```python
from build123d import *

# Parameters (mm, degrees)
SKETCH_1_W      = 1620
SKETCH_1_H      = 1620
SKETCH_1_W_2    = 500
SKETCH_1_H_2    = 500
EXTRUDE_1_DEPTH = 0.1


with BuildPart() as part:
    # 草图1 → 凸台-拉伸1 (new body)
    with BuildSketch(Plane(origin=(0, 0, 0), x_dir=(0, 0, -1), z_dir=(1, 0, 0))):
        Rectangle(SKETCH_1_W, SKETCH_1_H)
        with Locations((-540, 540)):
            Rectangle(SKETCH_1_W_2, SKETCH_1_H_2, mode=Mode.SUBTRACT)
        with Locations((0, 540)):
            Rectangle(SKETCH_1_W_2, SKETCH_1_H_2, mode=Mode.SUBTRACT)
        with Locations((540, 540)):
            Rectangle(SKETCH_1_W_2, SKETCH_1_H_2, mode=Mode.SUBTRACT)
        with Locations((540, 0)):
            Rectangle(SKETCH_1_W_2, SKETCH_1_H_2, mode=Mode.SUBTRACT)
        Rectangle(SKETCH_1_W_2, SKETCH_1_H_2, mode=Mode.SUBTRACT)
        with Locations((-540, 0)):
            Rectangle(SKETCH_1_W_2, SKETCH_1_H_2, mode=Mode.SUBTRACT)
        with Locations((-540, -540)):
            Rectangle(SKETCH_1_W_2, SKETCH_1_H_2, mode=Mode.SUBTRACT)
        with Locations((0, -540)):
            Rectangle(SKETCH_1_W_2, SKETCH_1_H_2, mode=Mode.SUBTRACT)
        with Locations((540, -540)):
            Rectangle(SKETCH_1_W_2, SKETCH_1_H_2, mode=Mode.SUBTRACT)
    extrude(amount=EXTRUDE_1_DEPTH)


solid = part.part
```
Source: CAD feature listing. Evaluate the final solid. Frame: model axes, mm. Round coordinates to 2 decimals unless told otherwise and drop trailing zeros. Order: outer loops, then holes, each group sorted by start corner. A loop starts at its lowest first (then second) coordinate and runs counter-clockwise, first axis right, second up. Notation, with made-up numbers: (53.5, 88) -> (92.5, 88) arc R23 ccw to (92.5, 104) -> close; hole circle Ø10 at (49.25, -29). An arc over 180 degrees is marked (long way). One line per item, written item: value. Start each with the question number.
Q1. Material intervals for probe 1 along Y at (x, z) = (0.05, 371), sorted ascending.
Q2. Section query C-C (x = 0.05). Give the number of separate pieces and of enclosed holes in the cut face, plus the area to 3 significant figures.
Q3. Section query A-A (z = 226). Return the cut outline in (x, y).
Findings below:
1. probe 1: -810 to -790, -290 to -250, 250 to 290, 790 to 810
2. separate pieces: 1
2. enclosed holes: 9
2. area: 374,000 mm²
3. outline: (0, -810) -> (0.1, -810) -> (0.1, -790) -> (0, -790) -> close; (0, -290) -> (0.1, -290) -> (0.1, -250) -> (0, -250) -> close; (0, 250) -> (0.1, 250) -> (0.1, 290) -> (0, 290) -> close; (0, 790) -> (0.1, 790) -> (0.1, 810) -> (0, 810) -> close
